Autodesk Inventor part; units mm, degrees
ref_plane "YZ Plane" through (0, 0, 0) normal (1, 0, 0) x (0, 1, 0)
ref_plane "XZ Plane" through (0, 0, 0) normal (0, 1, 0) x (-1, 0, 0)
ref_plane "XY Plane" through (0, 0, 0) normal (0, 0, 1) x (1, 0, 0)
sketch "Sketch4" plane through (0, 0, 0) normal (0, 1, 0) x (-1, 0, 0)
  line L0 (100, -60) -> (-100, -60)
  line L1 (-100, -60) -> (-100, 0)
  line L2 (-100, 0) -> (100, 0)
  line L3 (100, 0) -> (100, -60)
  point P0 (0, 0)
  point P1 (0, 0)
  dimension "d36" = 200
  dimension "d37" = 60
extrude "Plate2" add sketch "Sketch4" along normal blind 3
sketch "Sketch5" plane through (0, 0, 0) normal (0, -1, 0) x (1, 0, 0)
  circle A0 centre (-80, -30) radius 6.5
  circle A1 centre (80, -30) radius 6.5
  line L0 (0, 0) -> (0, -60) construction
  line L1 (100, -60) -> (-100, -60) construction
  line L2 (100, 0) -> (-100, 0)
  line L3 (80, -23.5) -> (-80, -23.5)
  line L4 (80, -36.5) -> (-80, -36.5)
  dimension "d39" = 160
  dimension "d40" = 30
  dimension "d41" = 13
  dimension "d55" = 60
extrude "Cut1" cut sketch "Sketch5" against normal blind 3
sketch "Sketch6" plane through (-100, 3, -3) normal (0, 0, 1) x (1, 0, 0)
  line L0 (200, 0) -> (0, 0)
  line L1 (0, 0) -> (0, -40)
  line L2 (0, -40) -> (200, -40)
  line L3 (200, -40) -> (200, 0)
edge flange "Flange1" height 40 angle 90 thickness 3 bend radius 5 thickness toward (0, 0, 1) relief round relief width 3 relief depth 1.5 corner gap 5 corner form 0 edges at (0, 0, 0) (0, 0, -60) wall of the first edge with corners at (100, 3, -3) (-100, 3, -3) (-100, -37, -3) (100, -37, -3)
bend "Bend1"
corner "Corner1"
equation "\"d40\" = 0.5 * d55"
equation "\"d42\" = Thickness"
equation "\"d38\" = Thickness"
equation "\"d44\" = BendReliefWidth"
equation "\"d45\" = BendReliefDepth"
equation "\"d46\" = MinimumRemnant"
equation "\"d47\" = TransitionRadius"
equation "\"d50\" = BendRadius"
equation "\"d51\" = CornerReliefSize"
equation "\"d52\" = GapSize"
equation "\"d53\" = JacobiRadiusSize"
equation "\"BendReliefWidth\" = Thickness"
equation "\"BendReliefDepth\" = 0.5 * Thickness"
equation "\"CornerReliefSize\" = 4 * Thickness"
equation "\"MinimumRemnant\" = 2 * Thickness"
equation "\"TransitionRadius\" = BendRadius"
equation "\"JacobiRadiusSize\" = BendRadius"
equation "\"GapSize\" = Thickness"
properties part number "NDM-VOS 715 flange" material "Stainless Steel"
Build history of the part. All positions in model axes, mm. A direction names the side the tool comes from. Round coordinates to 2 decimals unless told otherwise and drop trailing zeros. Loops run counter-clockwise (first coordinate to the right, second up) from the corner with the lowest first, then second, coordinate; pieces in that order, holes last.
Item 1: Pin check, flat tips, straight feed: P1, Ø22, axis at x = -49.5, z = -30, coming from the -Y side; P2, Ø1.5, axis at x = -13.5, y = 2, coming from the +Z side; P3, Ø3.5, axis at x = -19, y = 1, coming from the -Z side. Stop position of each tip, or through.
Item 2: Drill centre lines: line 1 along Z through (x, y) = (-47.5, -22); line 2 along Y through (x, z) = (-91.5, -22); line 3 along Z through (x, y) = (40.5, 0.5). Where is each one in solid material? Low to high.
Item 3: Saw through at A-A (x = 61). List the corners of the cut face in (y, z), then the cut area to 3 significant figures.
Item 4: Saw through at C-C (z = -30). List the corners of the cut face in (x, y).
Item 5: Which spindle directions (+Z, -Z, +X, -X, +Y, -Y) get a long thin tool onto all of the face, cutting with end or side? Do faces 1 (the face through (1, -2, -56)), 2 (the face through (100, 1, -30)), 3 (the face through (-86.5, 1.5, -29.9)). Say none if no direction does.
Item 6: Saw through at D-D (x = -84). List the corners of the cut face in (y, z).
Item 7: Saw through at B-B (y = -19). List the corners of the cut face in (x, z), then the cut area to 3 significant figures.
Item 8: Two-plate mould, pull along Z, no slides. Class faces 4 (the face through (1, 3, -39)), 5 (the face through (1, 0, -39)), 6 (the face through (1.4, 0.594, -57.719)): released by +Z, released by -Z, zero draft, split by the parting line, or undercut.
Worked answers:
1. P1: stops at y = 0
1. P2: stops at z = -3.01
1. P3: stops at z = -58.78
2. line 1: z = -60 to -57, -3 to 0
2. line 2: y = 0 to 3
2. line 3: z = -57.81 to -36.5, -23.5 to -2.19
3. outline: (-37, -60) - (-5, -60) arc R8 ccw to (3, -52) - (3, -36.5) - (0, -36.5) - (0, -52) arc R5 cw to (-5, -57) - (-37, -57) - close; (-37, -3) - (-5, -3) arc R5 cw to (0, -8) - (0, -23.5) - (3, -23.5) - (3, -8) arc R8 ccw to (-5, 0) - (-37, 0) - close
3. area: 346 mm2
4. outline: (-100, 0) - (-86.5, 0) - (-86.5, 3) - (-100, 3) - close; (86.5, 0) - (100, 0) - (100, 3) - (86.5, 3) - close
5. face 1: +X, -X, -Y
5. face 2: +Z, -Z, +X, +Y, -Y
5. face 3: +Y, -Y
6. outline: (-37, -60) - (-5, -60) arc R8 ccw to (3, -52) - (3, -35.12) - (0, -35.12) - (0, -52) arc R5 cw to (-5, -57) - (-37, -57) - close; (-37, -3) - (-5, -3) arc R5 cw to (0, -8) - (0, -24.88) - (3, -24.88) - (3, -8) arc R8 ccw to (-5, 0) - (-37, 0) - close
7. outline: (-100, -60) - (100, -60) - (100, -57) - (-100, -57) - close; (-100, -3) - (100, -3) - (100, 0) - (-100, 0) - close
7. area: 1,200 mm2
8. face 4: zero draft
8. face 5: undercut
8. face 6: released by -Z
